Autodesk Inventor part; units mm, degrees
ref_plane "YZ Plane" through (0, 0, 0) normal (1, 0, 0) x (0, 1, 0)
ref_plane "XZ Plane" through (0, 0, 0) normal (0, 1, 0) x (-1, 0, 0)
ref_plane "XY Plane" through (0, 0, 0) normal (0, 0, 1) x (1, 0, 0)
ref_plane "Work Plane1" through (0, 0, 0) normal (0, 0, 1) x (1, 0, 0)
sketch "Sketch1" plane through (0, 0, 0) normal (0, 0, 1) x (1, 0, 0)
  circle A0 centre (95.734, -21) radius 4.05
  circle A1 centre (170.734, -21) radius 4.05
  line L0 (78.234, -5) -> (78.234, 0)
  arc A2 (83.234, -10) -> (78.234, -5) centre (78.234, -10) ccw
  line L1 (83.234, -10) -> (83.234, -21)
  arc A3 (83.234, -21) -> (108.234, -21) centre (95.734, -21) ccw
  line L2 (108.234, -21) -> (108.234, -10)
  arc A4 (113.234, -5) -> (108.234, -10) centre (113.234, -10) ccw
  line L3 (113.234, -5) -> (153.234, -5)
  arc A5 (158.234, -10) -> (153.234, -5) centre (153.234, -10) ccw
  line L4 (158.234, -10) -> (158.234, -21)
  arc A6 (158.234, -21) -> (183.234, -21) centre (170.734, -21) ccw
  line L5 (183.234, -21) -> (183.234, -10)
  arc A7 (188.234, -5) -> (183.234, -10) centre (188.234, -10) ccw
  line L6 (188.234, 0) -> (188.234, -5)
  line L7 (78.234, 0) -> (188.234, 0)
  line L8 (437.5, 12.7) -> (437.5, 0)
  line L9 (0, 12.7) -> (437.5, 12.7)
  line L10 (0, 0) -> (0, 12.7)
  line L11 (437.5, 0) -> (0, 0)
  line L12 (0, 12.7) -> (0, -237.3)
  line L13 (0, -237.3) -> (25, -237.3)
  line L14 (25, -237.3) -> (180.7539, -28.4734)
  line L15 (183.234, -10) -> (183.234, 12.7)
  line L16 (183.234, 12.7) -> (0, 12.7)
  dimension "d0" = 25
  dimension "d2" = 250
extrude "Extrusion1" add sketch "Sketch1" along normal blind 12.7 contours A2 L1 A3 L2 A4 L3 A5 L4 A6 L14 L13 L12 L11 L0 | L0 L7 L15 L5 A6 L4 A5 L3 A4 L2 A3 L1 A2 | L11 L10 L9 L15 L7
properties part number "support"
Work out the finished part from the listing and answer in its coordinate system (mm). Round coordinates to 2 decimals unless told otherwise and drop trailing zeros. Loops run counter-clockwise (first coordinate to the right, second up) from the corner with the lowest first, then second, coordinate; pieces in that order, holes last. Notation, with made-up numbers: (25.5, 49.5) - (35.5, 49.5) arc R19 ccw to (35.5, 67.5) - close; hole circle Ø1 at (42.25, 78.25). An arc over 180 degrees is marked (long way). Use one line per item in the form item = value. Start each with the question number.
(1) Determine the mould class of faces 1 (the face through (91.69, -21.18, 6.26)), 2 (the face through (101.787, -134.348, 6.261)), 3 (the face through (70, -83, 12.7)) for opening direction X: +X half, -X half, draft (parallel to the pull), parting line (faces both ways), or undercut.
(2) Find section B-B on x = 78.5. Determine the outline of the cut face in (y, z), and give its area (3 significant figures).
(3) Find section A-A on z = 6. Determine the outline of the cut face in (x, y).
(4) Find section C-C on y = -112. Determine the outline of the cut face in (x, z), and give its area (3 significant figures).
(5) Consider line 1 (X direction, y = -24.5, z = 7); line 2 (X direction, y = -44.5, z = 8.25); line 3 (Y direction, x = 158, z = 4.75). Determine where each line is inside the solid, lowest interval first.
(6) Flat-ended cylindrical pins translate along their axes: P1, Ø2, axis at x = 29, z = 3, coming from the -Y side; P2, Ø6, axis at y = -52.5, z = 5.5, coming from the +X side. Find the tip coordinate at first contact, or state that the pin passes through.
Answer list:
q1.face_1 = undercut
q1.face_2 = +X half
q1.face_3 = draft
q2.outline = (-165.57, 0) - (12.7, 0) - (12.7, 12.7) - (-165.57, 12.7) - close
q2.area = 2,260 mm^2
q3.outline = (0, -237.3) - (25, -237.3) - (180.75, -28.47) arc R12.5 ccw to (183.23, -21) - (183.23, 12.7) - (0, 12.7) - close; hole circle Ø8.1 at (95.73, -21); hole circle Ø8.1 at (170.73, -21)
q4.outline = (0, 0) - (118.46, 0) - (118.46, 12.7) - (0, 12.7) - close
q4.area = 1,500 mm^2
q5.line_1 = 0 to 93.7, 97.77 to 168.7, 172.77 to 182.73
q5.line_2 = 0 to 168.8
q5.line_3 = -58.98 to 12.7
q6.P1 = -233.28
q6.P2 = 165.07
